CAD build for the part. Positions are in the model's coordinates, mm. Face numbers are marked on the shaded views. A direction names the side the tool comes from. Round coordinates to 2 decimals unless told otherwise and drop trailing zeros. Loops run counter-clockwise (first coordinate to the right, second up) from the corner with the lowest first, then second, coordinate; pieces in that order, holes last. Notation, with made-up numbers: M 37.25,4 L 67.25,4 A13 cw 67.25,20 Z; hole C -11.5,58.25 d9. An arc over 180 degrees is marked long. Use a Markdown table: item, result. Add a question column.
(1) Which spindle directions (+Z, -Z, +X, -X, +Y, -Y) get a long thin tool onto all of the face, cutting with end or side? Do the marked faces 1 and 2. Say none if no direction does.
(2) Wall check: L1, parallel to X at y = -41, z = 0; L2, parallel to Z at x = -71.5, y = 12.5; L3, parallel to Y at x = 275.5, z = 12. Give the ranges that are in metal, low to high.
(3) Band-saw the part on B-B, the plane x = -238.5. Write the cut outline in (y, z).
(4) Flat gauge pin, fed straight in: P1, Ø9, axis at x = 312.5, z = 0, coming from the -Y side. Where does the tip first touch, or does it go through?
(5) Two-plate mould, pull along Y, no slides. Class the marked faces 3 and 4: released by +Y, released by -Y, zero draft, split by the parting line, or undercut.
(6) Band-saw the part on C-C, the plane x = 350. Write the cut outline in (y, z).
(7) Band-saw the part on A-A, the plane y = 0. Give the number of separate pieces and of enclosed holes in the cut face, and give its area (3 significant figures).
from build123d import *

# Parameters (mm, degrees)
EXTRUDE_THIN1_DEPTH      = 420
EXTRUDE_THIN1_DEPTH_BACK = 420
CUT_EXTRUDE1_DEPTH       = 423.82147533
CUT_EXTRUDE1_DEPTH_BACK  = 423.82147533
SKETCH2_R                = 9
CUT_EXTRUDE2_DEPTH       = 423.82147533
CUT_EXTRUDE2_DEPTH_BACK  = 423.82147533
SKETCH3_R                = 5


with BuildPart() as part:
    # Sketch1 → Extrude-Thin1 (new, two sides: drawn at the far end of the back side and taken through both)
    with BuildSketch(Plane(origin=(0, 0, 0), x_dir=(0, 0, -1), z_dir=(1, 0, 0)).offset(-EXTRUDE_THIN1_DEPTH_BACK)):
        with BuildLine():
            Line((-23, 35), (-23, -35))
            ThreePointArc((-23, -35), (-20.656854249, -40.656854249), (-15, -43))
            Line((-15, -43), (15, -43))
            ThreePointArc((15, -43), (20.656854249, -40.656854249), (23, -35))
            Line((23, -35), (23, 35))
            ThreePointArc((23, 35), (20.656854249, 40.656854249), (15, 43))
            Line((15, 43), (-15, 43))
            ThreePointArc((-15, 43), (-20.656854249, 40.656854249), (-23, 35))
        make_face()
        with BuildLine():
            Line((-20, 35), (-20, -35))
            ThreePointArc((-20, -35), (-18.535533906, -38.535533906), (-15, -40))
            Line((-15, -40), (15, -40))
            ThreePointArc((15, -40), (18.535533906, -38.535533906), (20, -35))
            Line((20, -35), (20, 35))
            ThreePointArc((20, 35), (18.535533906, 38.535533906), (15, 40))
            Line((15, 40), (-15, 40))
            ThreePointArc((-15, 40), (-18.535533906, 38.535533906), (-20, 35))
        make_face(mode=Mode.SUBTRACT)
    extrude(amount=EXTRUDE_THIN1_DEPTH + EXTRUDE_THIN1_DEPTH_BACK)

    # Sketch2 → Cut-Extrude1 (cut, two sides: drawn at the far end of the back side and taken through both)
    with BuildSketch(Plane.XY.offset(-CUT_EXTRUDE1_DEPTH_BACK)):
        Circle(SKETCH2_R)
        with Locations((-350, 0)):
            Circle(SKETCH2_R)
        with Locations(Location((350, 0, 0), (0, 0, 180))):
            Circle(SKETCH2_R)
    extrude(amount=CUT_EXTRUDE1_DEPTH + CUT_EXTRUDE1_DEPTH_BACK, mode=Mode.SUBTRACT)

    # Sketch3 → Cut-Extrude2 (cut, two sides: drawn at the far end of the back side and taken through both)
    with BuildSketch(Plane(origin=(0, 0, 0), x_dir=(1, 0, 0), z_dir=(0, 1, 0)).offset(-CUT_EXTRUDE2_DEPTH_BACK)):
        with Locations(Location((-387.5, 0, 0), (0, 0, 270))):
            Circle(SKETCH3_R)
        with Locations(Location((-312.5, 0, 0), (0, 0, 270))):
            Circle(SKETCH3_R)
        with Locations(Location((312.5, 0, 0), (0, 0, 90))):
            Circle(SKETCH3_R)
        with Locations(Location((387.5, 0, 0), (0, 0, 90))):
            Circle(SKETCH3_R)
    extrude(amount=CUT_EXTRUDE2_DEPTH + CUT_EXTRUDE2_DEPTH_BACK, mode=Mode.SUBTRACT)


solid = part.part
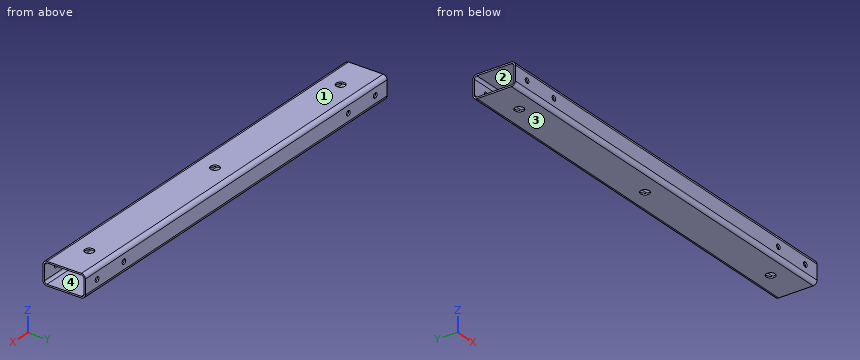
Return value:
| question | item | result |
|---|---|---|
| 1 | face 1 | +Z, +X, -X, +Y, -Y |
| 1 | face 2 | +X, -X |
| 2 | L1 | -420 to -392.5, -382.5 to -317.5, -307.5 to 307.5, 317.5 to 382.5, 392.5 to 420 |
| 2 | L2 | -23 to -20, 20 to 23 |
| 2 | L3 | -43 to -40, 40 to 43 |
| 3 | outline | M -43,-15 A8 ccw -35,-23 L 35,-23 A8 ccw 43,-15 L 43,15 A8 ccw 35,23 L -35,23 A8 ccw -43,15 Z; hole M -40,-15 A5 ccw -35,-20 L 35,-20 A5 ccw 40,-15 L 40,15 A5 ccw 35,20 L -35,20 A5 ccw -40,15 Z |
| 4 | P1 | through |
| 5 | face 3 | zero draft |
| 5 | face 4 | undercut |
| 6 | outline | M -43,-15 A8 ccw -35,-23 L -9,-23 L -9,-20 L -35,-20 A5 cw -40,-15 L -40,15 A5 cw -35,20 L -9,20 L -9,23 L -35,23 A8 ccw -43,15 Z; M 9,-23 L 35,-23 A8 ccw 43,-15 L 43,15 A8 ccw 35,23 L 9,23 L 9,20 L 35,20 A5 cw 40,15 L 40,-15 A5 cw 35,-20 L 9,-20 Z |
| 7 | separate pieces | 8 |
| 7 | enclosed holes | 0 |
| 7 | area | 4,720 mm^2 |
